```python
from build123d import *

# Parameters (mm, degrees)
BOSS_EXTRUDE1_DEPTH = 5
CUT_EXTRUDE1_DEPTH  = 10
FILLET1_R           = 0.5


with BuildPart() as part:
    # Sketch1 → Boss-Extrude1 (new body)
    with BuildSketch(Plane(origin=(0, 0, 0), x_dir=(1, 0, 0), z_dir=(0, 1, 0))):
        with BuildLine():
            Line((-1.5, 4.588107716), (-0.821593865, 2.908993609))
            ThreePointArc((-0.821593865, 2.908993609), (-1.925604645, 2.412618737), (-2.771400023, 1.546675324))
            Line((-2.771400023, 1.546675324), (-4.18358485, 2.731639091))
            Line((-4.18358485, 2.731639091), (-5.110635833, -0.121530457))
            Line((-5.110635833, -0.121530457), (-3.304064395, 0.004797324))
            ThreePointArc((-3.304064395, 0.004797324), (-3.173141931, -1.198567594), (-2.610945952, -2.27055803))
            Line((-2.610945952, -2.27055803), (-4.174302575, -3.24745167))
            Line((-4.174302575, -3.24745167), (-1.747251592, -5.010807427))
            Line((-1.747251592, -5.010807427), (-1.309135176, -3.253618458))
            ThreePointArc((-1.309135176, -3.253618458), (-0.124209863, -3.500964005), (1.069041739, -3.297547119))
            Line((1.069041739, -3.297547119), (1.515019036, -5.086264359))
            Line((1.515019036, -5.086264359), (3.942070019, -3.322908602))
            Line((3.942070019, -3.322908602), (2.406269417, -2.363233875))
            ThreePointArc((2.406269417, -2.363233875), (3.007671071, -1.312736913), (3.182945139, -0.115027927))
            Line((3.182945139, -0.115027927), (5.02193089, -0.243622337))
            Line((5.02193089, -0.243622337), (4.094879907, 2.609547212))
            Line((4.094879907, 2.609547212), (2.707586519, 1.445469841))
            ThreePointArc((2.707586519, 1.445469841), (1.894347869, 2.342058217), (0.809421598, 2.878866192))
            Line((0.809421598, 2.878866192), (1.5, 4.588107716))
            Line((1.5, 4.588107716), (-1.5, 4.588107716))
        make_face()
    extrude(amount=BOSS_EXTRUDE1_DEPTH)

    # Sketch2 → Cut-Extrude1 (cut)
    with BuildSketch(Plane(origin=(0, 5, 0), x_dir=(1, 0, 0), z_dir=(0, 1, 0))):
        with BuildLine():
            Line((-1.25, 0), (-2.5, 0))
            ThreePointArc((-2.5, 0), (0, -2.5), (2.5, 0))
            Line((2.5, 0), (1.25, 0))
            ThreePointArc((1.25, 0), (0, 1.25), (-1.25, 0))
        make_face()
    extrude(amount=-CUT_EXTRUDE1_DEPTH, mode=Mode.SUBTRACT)

    # Fillet1
    fillet1_edges = [part.edges().sort_by_distance(p)[0] for p in [
        (3.942070019, 2.5, 3.322908602),
        (1.515019036, 2.5, 5.086264359),
        (-1.747251592, 2.5, 5.010807427),
        (-4.174302575, 2.5, 3.24745167),
        (-5.110635833, 2.5, 0.121530457),
        (-4.18358485, 2.5, -2.731639091),
        (-1.5, 2.5, -4.588107716),
        (1.5, 2.5, -4.588107716),
        (4.094879907, 2.5, -2.609547212),
        (5.02193089, 2.5, 0.243622337),
    ]]
    fillet(fillet1_edges, radius=FILLET1_R)


solid = part.part
```
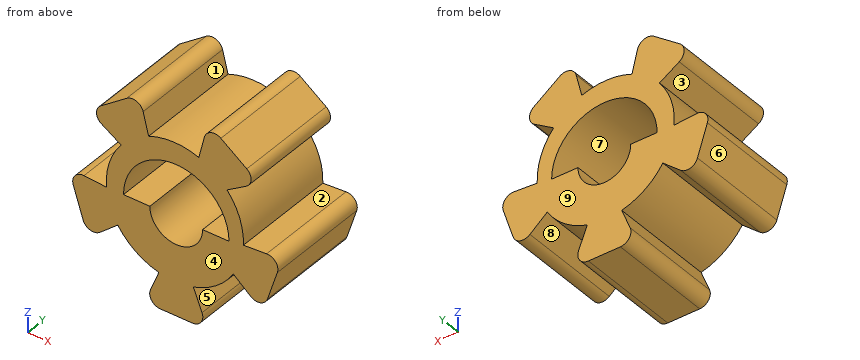
Verification items for the finished model (mm, model axes). Face numbers are marked on the shaded views. A direction names the side the tool comes from. Coordinates: 2 decimals unless noted, no trailing zeros. Loops run counter-clockwise (first coordinate to the right, second up) from the corner with the lowest first, then second, coordinate; pieces in that order, holes last. Notation, with made-up numbers: (0, 76.25) - (28, 76.25) arc R33 ccw to (28, 113.25) - close; hole circle Ø6 at (14, 74.25). An arc over 180 degrees is marked (long way). Return JSON: item names as keys, results as strings.
1. Thickness scan on L1, parallel to X at y = 1.5, z = -2; L2, parallel to Z at x = -0.5, y = 0.85; L3, parallel to Z at x = -1.75, y = 2.9. Record the ranges inside material, lowest first.
Established:
{"L1": "x = -4.42 to -3.31, -2.41 to 2.28, 3.37 to 4.28", "L2": "z = -4.59 to -1.15, 2.45 to 3.47", "L3": "z = -2.53 to 0, 1.79 to 4.57"}
2. Section check D-D, the plane z = 4. Record the boundary of the cut face in (x, y), then the cut area to 3 significant figures.
Established:
{"outline": "(-3.14, 0) - (-1.5, 0) - (-1.5, 5) - (-3.14, 5) - close; (1.24, 0) - (3.01, 0) - (3.01, 5) - (1.24, 5) - close", "area": "17.0 mm2"}
3. Go/stop test with flat-tipped pins: pin 1 (3 mm diameter, centred on x = -3, y = 1.5, fed in from -Z); pin 2 (2 mm diameter, centred on x = -1, y = 1.5, fed in from +Z); pin 3 (1.5 mm diameter, centred on x = -3.5, y = 4, fed in from +Z). Record where each tip stops, or that it passes through.
Established:
{"pin 1": "stops at z = -2.66", "pin 2": "stops at z = 4.67", "pin 3": "stops at z = 4.28"}
4. Section check B-B, the plane x = -0.25. Record the boundary of the cut face in (y, z), then the cut area to 3 significant figures.
Established:
{"outline": "(0, -4.59) - (5, -4.59) - (5, -1.22) - (0, -1.22) - close; (0, 2.49) - (5, 2.49) - (5, 3.5) - (0, 3.5) - close", "area": "21.9 mm2"}
5. Mould release check, pull along X, two halves, no side actions. Record for the marked faces 6, 7, 8 and 9: +X half, -X half, draft (parallel to the pull), parting line (faces both ways), or undercut.
Established:
{"face 6": "-X half", "face 7": "undercut", "face 8": "undercut", "face 9": "draft"}
6. Tool access check on the marked faces 1, 2, 3, 4 and 5. Record the directions out of +Z, -Z, +X, -X, +Y, -Y that give a thin tool (end or side, any length) a straight path to the whole face; none if there is none.
Established:
{"face 1": "+Z, +Y, -Y", "face 2": "+Y, -Y", "face 3": "-X, +Y, -Y", "face 4": "+Z, -Z, +X, -X, -Y", "face 5": "+X, +Y, -Y"}
7. Section check C-C, the plane z = -1.75. Record the boundary of the cut face in (x, y), then the cut area to 3 significant figures.
Established:
{"outline": "(-4.5, 0) - (-3.01, 0) - (-3.01, 5) - (-4.5, 5) - close; (-2.62, 0) - (2.5, 0) - (2.5, 5) - (-2.62, 5) - close; (3.07, 0) - (4.37, 0) - (4.37, 5) - (3.07, 5) - close", "area": "39.6 mm2"}
